Verification items for this drawing (mm, ordinates from the low corner). A direction names the side the tool comes from. Coordinates: 2 decimals unless noted, no trailing zeros. Loops run counter-clockwise (first coordinate to the right, second up) from the corner with the lowest first, then second, coordinate; pieces in that order, holes last. Notation, with made-up numbers: (-9.5, 17) -> (-4.5, 17) arc R16 cw to (-4.5, 47) -> close; hole circle Ø6 at (-29, -23). An arc over 180 degrees is marked (long way). Write item = value, one per line.
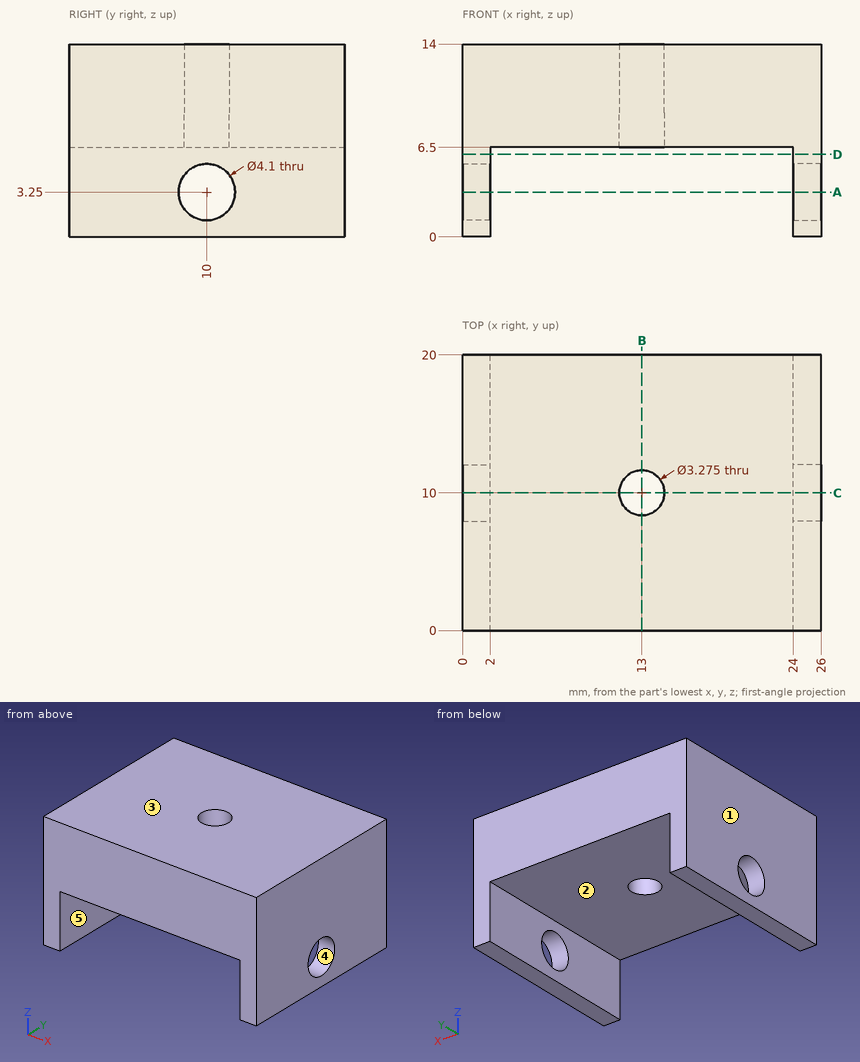
1) Tool access check on the marked faces 1 and 2. Record the directions out of +Z, -Z, +X, -X, +Y, -Y that give a thin tool (end or side, any length) a straight path to the whole face; none if there is none.
Ans:
face_1 = +Z, -Z, -X, +Y, -Y
face_2 = -Z, +Y, -Y
2) Material ranges on line 1 (Z direction, x = 25.65, y = 10); line 2 (Y direction, x = 13, z = 10.6); line 3 (X direction, y = 8.75, z = 6), recorded low to high.
Ans:
line_1 = 0 to 1.2, 5.3 to 14
line_2 = 0 to 8.36, 11.64 to 20
line_3 = 0 to 2, 24 to 26
3) Depth check by flat-ended pin: pin 1 Ø5 at (x, z) = (14.5, 2) entering from +Y; pin 2 Ø1.5 at (x, y) = (19, 12.5) entering from -Z. Enter the tip coordinate at first touch or a pass-through.
Ans:
pin_1 = through
pin_2 = 6.5
4) Sectioned sample at A-A, the plane z = 3.25. Record the cut outline in (x, y), plus the area to 3 significant figures.
Ans:
outline = (0, 0) -> (2, 0) -> (2, 7.95) -> (0, 7.95) -> close; (0, 12.05) -> (2, 12.05) -> (2, 20) -> (0, 20) -> close; (24, 0) -> (26, 0) -> (26, 7.95) -> (24, 7.95) -> close; (24, 12.05) -> (26, 12.05) -> (26, 20) -> (24, 20) -> close
area = 63.6 mm2
5) Sectioned sample at C-C, the plane y = 10. Record the cut outline in (x, z), plus the area to 3 significant figures.
Ans:
outline = (0, 0) -> (2, 0) -> (2, 1.2) -> (0, 1.2) -> close; (0, 5.3) -> (2, 5.3) -> (2, 6.5) -> (11.36, 6.5) -> (11.36, 14) -> (0, 14) -> close; (14.64, 6.5) -> (24, 6.5) -> (24, 5.3) -> (26, 5.3) -> (26, 14) -> (14.64, 14) -> close; (24, 0) -> (26, 0) -> (26, 1.2) -> (24, 1.2) -> close
area = 180 mm2
6) Release check for a two-part mould opening along Z. For the marked faces 3, 4 and 5 record: pulls with the +Z half, pulls with the -Z half, needs draft (parallel to the pull), parting line crosses it, or undercut.
Ans:
face_3 = pulls with the +Z half
face_4 = undercut
face_5 = needs draft
7) Sectioned sample at B-B, the plane x = 13. Record the cut outline in (y, z), plus the area to 3 significant figures.
Ans:
outline = (0, 6.5) -> (8.36, 6.5) -> (8.36, 14) -> (0, 14) -> close; (11.64, 6.5) -> (20, 6.5) -> (20, 14) -> (11.64, 14) -> close
area = 125 mm2
8) Sectioned sample at D-D, the plane z = 6. Record the cut outline in (x, y), plus the area to 3 significant figures.
Ans:
outline = (0, 0) -> (2, 0) -> (2, 20) -> (0, 20) -> close; (24, 0) -> (26, 0) -> (26, 20) -> (24, 20) -> close
area = 80.0 mm2
